Verification items for this drawing (mm, ordinates from the low corner). A direction names the side the tool comes from. Round coordinates to 2 decimals unless told otherwise and drop trailing zeros. Loops run counter-clockwise (first coordinate to the right, second up) from the corner with the lowest first, then second, coordinate; pieces in that order, holes last. Notation, with made-up numbers: (69, -33.5) -> (93, -33.5) arc R17 cw to (93, -22.5) -> close; hole circle Ø7 at (32.25, 36). An arc over 180 degrees is marked (long way). Use a Markdown table: item, result. Add a question column.
Q1. Sectioned sample at B-B, the plane x = 143. Enter the section's corners in (y, z) (1 decimal).
Q2. Set-up check for the marked faces 1, 2, 3, 4 and 5: record each of +Z, -Z, +X, -X, +Y, -Y from which the full face is reachable in a straight line by a thin tool's end or side.
Q3. Gauge pin test, flat ends, axial feed: P1, Ø12, axis at x = 126, z = 44.5, coming from the -Y side; P2, Ø8, axis at y = 8.5, z = 35, coming from the -X side; P3, Ø12, axis at x = 64, z = 38.5, coming from the -Y side. Record the tip position at first contact, or that the pin passes through.
Q4. Material ranges on L1, parallel to X at y = 11.5, z = 34.5; L2, parallel to Z at x = 84.5, y = 12; L3, parallel to Z at x = 57.5, y = 16, recorded low to high.
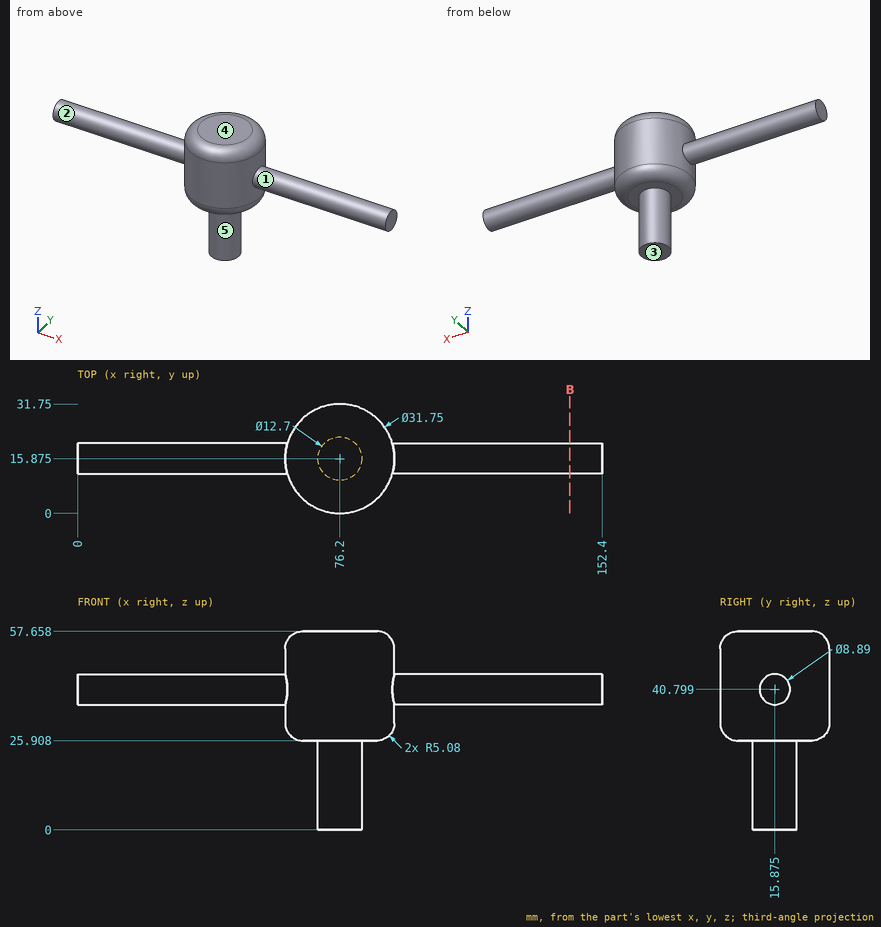
Values:
| question | item | result |
|---|---|---|
| 1 | outline | circle Ø8.9 at (15.9, 40.8) |
| 2 | face 1 | +X |
| 2 | face 2 | -X |
| 2 | face 3 | -Z, +X, -X, +Y, -Y |
| 2 | face 4 | +Z, +X, -X, +Y, -Y |
| 2 | face 5 | -Z |
| 3 | P1 | y = 11.43 |
| 3 | P2 | x = 60.69 |
| 3 | P3 | y = 1.26 |
| 4 | L1 | 60.94 to 91.46 |
| 4 | L2 | 25.91 to 57.66 |
| 4 | L3 | 36.36 to 45.24 |
